Model file for the job. Use its own axes, mm. Face numbers are marked on the shaded views. A direction names the side the tool comes from. Give positions to 0.01 mm unless a question says otherwise; leave off trailing zeros. Loops run counter-clockwise (first coordinate to the right, second up) from the corner with the lowest first, then second, coordinate; pieces in that order, holes last. Notation, with made-up numbers: (25.5, -14.5) -> (37.5, -14.5) arc R33 cw to (37.5, 13.5) -> close; hole circle Ø1 at (-32, 0.25). An arc over 180 degrees is marked (long way). Use CSV: the item, a comma, the result in double quotes. Start each with the question number.
(1) Flat gauge pins, fed straight in: pin 1 (5 mm diameter, centred on x = -4.5, z = 20.5, fed in from +Y); pin 2 (6 mm diameter, centred on x = -5, z = 24, fed in from +Y); pin 3 (1.5 mm diameter, centred on y = -1, z = 11, fed in from +X); pin 4 (1 mm diameter, centred on x = -4.5, z = 30, fed in from -Y). Where does each tip first touch, or does it go through?
(2) Cut at C-C on z = 30. Write the cut outline in (x, y), then the cut area to 3 significant figures.
(3) 3-axis set-ups, long thin cutter, end or side, ignore diameter. For the marked faces 1, 2, 3 and 4: which of +Z, -Z, +X, -X, +Y, -Y reach the whole face in a straight line?
(4) Cut at B-B on y = -3.95. Write the cut outline in (x, z), then the cut area to 3 significant figures.
(5) Cut at A-A on x = -13. Write the cut outline in (y, z).
(6) Drill centre lines: probe 1 along X at (y, z) = (-2.9, 5.5); probe 2 along Z at (x, y) = (-13, -2.25); probe 3 along Y at (x, z) = (-10.5, 15). Where is each one in solid material? Low to high.
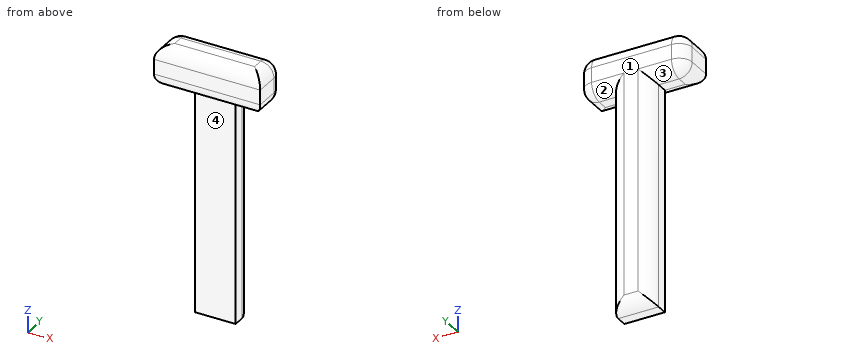
from build123d import *

# Parameters (mm, degrees)
F0_W     = 5.288299
F0_H     = 29.085644
F1_DEPTH = 3.10534
F3_DEPTH = 4.83128
F4_R     = 1.714961


with BuildPart() as f1:
    # F0 (on Front) → F1 (new body)
    with BuildSketch(Plane.XZ):
        with Locations((-9.695214, 14.542822)):
            Rectangle(F0_W, F0_H)
    extrude(amount=F1_DEPTH)

    # F2 (on Front) → F3 (join)
    with BuildSketch(Plane.XZ):
        Polygon((-16.712353, 29.071761), (-12.286842, 29.071761), (-7.046107, 29.071761), (-2.853518, 29.071761), (-2.853518, 34.428958), (-16.712353, 34.428958), align=None)
    extrude(amount=F3_DEPTH)

    # F4
    f4_edges = [f1.edges().sort_by_distance(p)[0] for p in [
        (-16.712353, -2.41564, 34.428958),
        (-16.712353, -2.41564, 29.071761),
        (-2.853518, -2.41564, 34.428958),
        (-9.782935, -4.83128, 29.071761),
        (-2.853518, -2.41564, 29.071761),
        (-9.782935, -4.83128, 34.428958),
        (-16.712353, 0, 31.75036),
        (-14.525858, 0, 29.071761),
        (-12.339364, 0, 14.535881),
        (-9.695214, 0, 0),
        (-7.051065, 0, 14.535881),
        (-4.952291, 0, 29.071761),
        (-2.853518, 0, 31.75036),
        (-9.782935, 0, 34.428958),
    ]]
    fillet(f4_edges, radius=F4_R)


solid = f1.part
Check result:
1,pin 1,"through"
1,pin 2,"y = -0.18"
1,pin 3,"x = -7.05"
1,pin 4,"y = -4.81"
2,outline,"(-16.52, -4.64) -> (-3.04, -4.64) -> (-3.04, -1.71) arc R1.52 ccw to (-4.57, -0.19) -> (-7.98, -0.19) arc R1.71 ccw to (-8.77, 0) -> (-10.62, 0) arc R1.71 ccw to (-11.41, -0.19) -> (-15, -0.19) arc R1.52 ccw to (-16.52, -1.71) -> close"
2,area,"59.5 mm²"
3,face 1,"+Z, -Z, +X, -X, +Y"
3,face 2,"-Z, +X, +Y"
3,face 3,"-Z, -X, +Y"
3,face 4,"-Z, +X, -X, -Y"
4,outline,"(-16.71, 30.79) arc R1.71 ccw to (-15.83, 29.29) -> (-3.73, 29.29) arc R1.71 ccw to (-2.85, 30.79) -> (-2.85, 32.71) arc R1.71 ccw to (-3.73, 34.21) -> (-15.83, 34.21) arc R1.71 ccw to (-16.71, 32.71) -> close"
4,area,"66.7 mm²"
5,outline,"(-4.83, 30.79) arc R1.71 ccw to (-3.12, 29.07) -> (-1.71, 29.07) arc R1.71 ccw to (0, 30.79) -> (0, 32.71) arc R1.71 ccw to (-1.71, 34.43) -> (-3.12, 34.43) arc R1.71 ccw to (-4.83, 32.71) -> close"
6,probe 1,"-12.34 to -7.05"
6,probe 2,"29.07 to 34.43"
6,probe 3,"-3.11 to 0"
